Part model, mm, in its own coordinate system. A direction names the side the tool comes from. Coordinates: 2 decimals unless noted, no trailing zeros. Order: outer loops, then holes, each group sorted by start corner. A loop starts at its lowest first (then second) coordinate and runs counter-clockwise, first axis right, second up.
1) Pin check, flat tips, straight feed: pin 1 Ø4 at (x, z) = (2.5, 1.5) entering from -Y; pin 2 Ø1 at (x, y) = (-4, -18) entering from +Z; pin 3 Ø1.2 at (x, y) = (0.5, -0.5) entering from -Z. Stop position of each tip, or through.
2) Wall check: L1, parallel to Y at x = 0, z = -3.5; L2, parallel to Z at x = 5, y = -24; L3, parallel to Y at x = -1.5, z = -7. Give the ranges that are in metal, low to high.
3) Cut at C-C (z = -7.5). List the corners of the cut face in (x, y).
4) Cut at B-B (y = 0). List the corners of the cut face in (x, z), and give its area (3 significant figures).
5) Tool access for faces 1 (the flat face through (0, 0, 5.6)), 2 (the flat face through (0, -35, -12)), 3 (the flat face through (0, -35, 0)), 4 (the cylindrical face through (0, -2, -8)), 5 (the flat face through (0, 3.5, -5)): list every direction of +Z, -Z, +X, -X, +Y, -Y with a clear straight run to the whole face (end or side of a thin tool).
6) Cut at D-D (x = 3.5). List the corners of the cut face in (y, z), and give its area (3 significant figures).
7) Mould opens along X. For faces 6 (the cylindrical face through (-6.9, 2.93, -5.05)), 7 (the flat face through (2, -2, -16)), 8 (the flat face through (0, 0, 0)) say: +X half, -X half, draft (parallel to the pull), parting line (faces both ways), or undercut.
8) Cut at A-A (x = 0). List the corners of the cut face in (y, z).
Autodesk Inventor part; units mm, degrees
ref_plane "YZ Plane" through (0, 0, 0) normal (1, 0, 0) x (0, 1, 0)
ref_plane "XZ Plane" through (0, 0, 0) normal (0, 1, 0) x (-1, 0, 0)
ref_plane "XY Plane" through (0, 0, 0) normal (0, 0, 1) x (1, 0, 0)
sketch "Sketch1" plane through (0, 0, 0) normal (0, 0, 1) x (1, 0, 0)
  circle A0 centre (0, 0) radius 2
  line L0 (-5.5, 3.5) -> (5.5, 3.5)
  line L1 (7.5, 1.5) -> (7.5, -3.5)
  line L2 (7.5, -3.5) -> (-7.5, -3.5)
  line L3 (-7.5, -3.5) -> (-7.5, 1.5)
  arc A1 (-5.5, 3.5) -> (-7.5, 1.5) centre (-5.5, 1.5) ccw
  arc A2 (7.5, 1.5) -> (5.5, 3.5) centre (5.5, 1.5) ccw
  point P0 (7.5, 3.5)
  dimension "d0" = 4
  dimension "d1" = 15
  dimension "d2" = 7
  dimension "d3" = 7.5
  dimension "d4" = 3.5
  dimension "d5" = 2
extrude "Extrusion1" add sketch "Sketch1" against normal blind 16
sketch "Sketch2" plane through (-7.5, -3.5, 0) normal (0, -1, 0) x (-1, 0, 0)
  line L0 (-15, 0) -> (-13, 0)
  line L1 (0, 12) -> (-15, 12)
  line L2 (-15, 12) -> (-15, 0)
  line L3 (-15, 0) -> (0, 0)
  line L4 (0, 0) -> (0, 12)
  line L5 (-15, 16) -> (0, 16)
  line L6 (0, 0) -> (0, 16)
  point P0 (-7.5, 0)
  dimension "d8" = 4
  dimension "d9" = 0
  dimension "d18" = 15
  dimension "d19" = 12
extrude "Extrusion2" add sketch "Sketch2" along normal blind 55.5
fillet "Fillet2" radius 10 1 edges at (0, -3.5, -12)
sketch "Sketch4" plane through (0, 0, 0) normal (0, 0, 1) x (1, 0, 0)
  line L0 (7.5, -3.5) -> (-7.5, -3.5)
  line L1 (7.5, -3.5) -> (-7.5, -3.5)
  line L2 (-7.5, -3.5) -> (-7.5, 1.5)
  line L3 (-5.5, 3.5) -> (5.5, 3.5)
  line L4 (7.5, 1.5) -> (7.5, -3.5)
  arc A0 (-5.5, 3.5) -> (-7.5, 1.5) centre (-5.5, 1.5) ccw
  arc A1 (7.5, 1.5) -> (5.5, 3.5) centre (5.5, 1.5) ccw
  point P0 (0, 0)
  dimension "d14" = 2
extrude "Extrusion3" add sketch "Sketch4" along normal blind 5.6
fillet "Fillet3" radius 10 1 edges at (0, -3.5, 0)
properties part number "frontside arm" material "UHMW, Black"
Geometry check:
1. pin 1: stops at y = -59
1. pin 2: stops at z = 0
1. pin 3: stops at z = 0
2. L1: y = -59 to -2, 2 to 3.5
2. L2: z = -12 to 0
2. L3: y = -59 to -1.32, 1.32 to 3.5
3. outline: (-7.5, -59) - (7.5, -59) - (7.5, 1.5) arc R2 ccw to (5.5, 3.5) - (-5.5, 3.5) arc R2 ccw to (-7.5, 1.5) - close; hole circle Ø4 at (0, 0)
4. outline: (-7.5, -16) - (-2, -16) - (-2, 0) - (2, 0) - (2, -16) - (7.5, -16) - (7.5, 5.6) - (-7.5, 5.6) - close
4. area: 260 mm2
5. face 1: +Z, +X, -X, +Y, -Y
5. face 2: -Z, +X, -X, -Y
5. face 3: +Z, +X, -X, -Y
5. face 4: -Z
5. face 5: +Z, -Z, +X, -X, +Y
6. outline: (-59, -12) - (-11.5, -12) arc R10 cw to (-3.5, -16) - (3.5, -16) - (3.5, 5.6) - (-3.5, 5.6) arc R10 cw to (-12.48, 0) - (-59, 0) - close
6. area: 841 mm2
7. face 6: -X half
7. face 7: draft
7. face 8: undercut
8. outline: (-59, -12) - (-11.5, -12) arc R10 cw to (-3.5, -16) - (-2, -16) - (-2, 0) - (2, 0) - (2, -16) - (3.5, -16) - (3.5, 5.6) - (-3.5, 5.6) arc R10 cw to (-12.48, 0) - (-59, 0) - close
